```python
from build123d import *

# Parameters (mm, degrees)
BOSS_EXTRUDE1_DEPTH                           = 30
SKETCH2_R                                     = 3.2639
CUT_EXTRUDE1_DEPTH                            = 36
CBORE_FOR_1_4_SOCKET_HEAD_CAP_SCREW1_AT_COUNT = 2
CBORE_FOR_1_4_SOCKET_HEAD_CAP_SCREW1_AT_PITCH = 35
SKETCH7_W                                     = 15
SKETCH7_H                                     = 6.5
BOSS_EXTRUDE2_DEPTH                           = 3
FILLET1_R                                     = 2
CHAMFER1_SIZE                                 = 0.2


with BuildPart() as part:
    # Sketch1 → Boss-Extrude1 (new body)
    with BuildSketch(Plane.XY):
        Polygon((20, 0), (0, 0), (0, 50.45), (-15, 50.45), (-15, 0), (-35, 0), (-35, -20), (20, -20), align=None)
    extrude(amount=BOSS_EXTRUDE1_DEPTH)

    # Sketch2 → Cut-Extrude1 (cut, through all)
    with BuildSketch(Plane(origin=(0, 0, 0), x_dir=(0, 0, -1), z_dir=(1, 0, 0))):
        with Locations((-15, 40.45)):
            Circle(SKETCH2_R)
    extrude(amount=-CUT_EXTRUDE1_DEPTH, mode=Mode.SUBTRACT)

    # Sketch5 → CBORE for 1/4 Socket Head Cap Screw1 (revolve, cut)
    with BuildSketch(Plane(origin=(-25, 0, 15), x_dir=(0, 0, 1), z_dir=(1, 0, 0))):
        Polygon((0, 0), (0, 20), (3.8989, 20), (3.2639, 19.365), (3.2639, 7.984998), (3.8989, 7.349998), (5.55625, 7.349998), (5.55625, 0.635), (6.19125, 0), align=None)
    cbore_for_1_4_socket_head_cap_screw1 = revolve(axis=Axis((-25, 6.35, 15), (0, -1, 0)), mode=Mode.SUBTRACT)

    # CBORE for 1/4 Socket Head Cap Screw1 at: CBORE for 1/4 Socket Head Cap Screw1 ×2
    with Locations(*[(i * CBORE_FOR_1_4_SOCKET_HEAD_CAP_SCREW1_AT_PITCH, 0, 0) for i in range(1, CBORE_FOR_1_4_SOCKET_HEAD_CAP_SCREW1_AT_COUNT)]):
        add(cbore_for_1_4_socket_head_cap_screw1, mode=Mode.SUBTRACT)

    # Sketch7 → Boss-Extrude2 (add)
    with BuildSketch(Plane.XZ.offset(20)):
        with Locations((-7.5, 15)):
            Rectangle(SKETCH7_W, SKETCH7_H)
    extrude(amount=BOSS_EXTRUDE2_DEPTH)

    # Fillet1
    fillet1_edges = [part.edges().sort_by_distance(p)[0] for p in [
        (-35, -10, 30),
        (-15, 25.225, 0),
        (-7.5, 50.45, 0),
        (0, 25.225, 0),
        (10, 0, 0),
        (20, -10, 0),
        (-35, -10, 0),
        (-25, 0, 0),
        (-15, 50.45, 15),
        (0, 50.45, 15),
        (20, 0, 15),
        (-35, 0, 15),
        (20, -10, 30),
        (10, 0, 30),
        (0, 25.225, 30),
        (-7.5, 50.45, 30),
        (-15, 25.225, 30),
        (-25, 0, 30),
        (-15, -21.5, 11.75),
        (0, -21.5, 11.75),
        (0, -21.5, 18.25),
        (-15, -21.5, 18.25),
    ]]
    fillet(fillet1_edges, radius=FILLET1_R)

    # Chamfer1
    chamfer1_edges = [part.edges().sort_by_distance(p)[0] for p in [
        (-35, -20, 15),
        (-34.414213562, -20, 29.414213562),
        (-34.414213562, -20, 0.585786438),
        (19.414213562, -20, 0.585786438),
        (19.414213562, -20, 29.414213562),
        (-15, 40.45, 18.2639),
        (0, 40.45, 18.2639),
        (0, -23, 15),
        (-7.5, -23, 11.75),
        (-7.5, -23, 18.25),
        (-15, -23, 15),
        (-14.414213562, -23, 12.335786438),
        (-14.414213562, -23, 17.664213562),
        (-0.585786438, -23, 17.664213562),
        (-0.585786438, -23, 12.335786438),
        (-7.5, -20, 0),
        (-7.5, -20, 30),
        (20, -20, 15),
    ]]
    chamfer(chamfer1_edges, length=CHAMFER1_SIZE)


solid = part.part
```
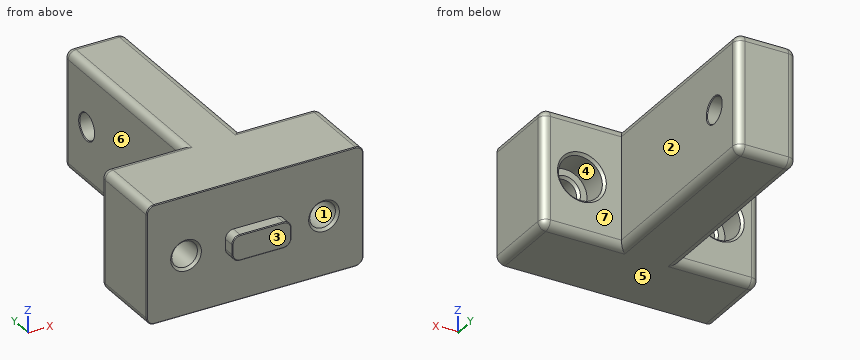
Verification items for the finished model (mm, model axes). Face numbers are marked on the shaded views. A direction names the side the tool comes from. Give positions to 0.01 mm unless a question says otherwise; leave off trailing zeros. Order: outer loops, then holes, each group sorted by start corner. A loop starts at its lowest first (then second) coordinate and runs counter-clockwise, first axis right, second up. Notation, with made-up numbers: (54.25, 74.25) -> (90.25, 74.25) arc R10 cw to (90.25, 90.25) -> close; hole circle Ø5 at (64, 25). An arc over 180 degrees is marked (long way). Use a Markdown table: item, result.
1) Section check C-C, the plane x = -17.5. Record the boundary of the cut face in (y, z), then the cut area to 3 significant figures.
Results:
| item | result |
|---|---|
| outline | (-20, 0.2) -> (-19.8, 0) -> (-2, 0) arc R2 ccw to (0, 2) -> (0, 28) arc R2 ccw to (-2, 30) -> (-19.8, 30) -> (-20, 29.8) -> close |
| area | 598 mm² |
2) Material ranges on probe 1 along X at (y, z) = (-3.5, 15); probe 2 along X at (y, z) = (-11, 14.75); probe 3 along Z at (x, y) = (10, -3), recorded low to high.
Results:
| item | result |
|---|---|
| probe 1 | -35 to -30.56, -19.44 to 4.44, 15.56 to 20 |
| probe 2 | -35 to -28.25, -21.75 to 6.75, 13.25 to 20 |
| probe 3 | 0 to 9.44, 20.56 to 30 |
3) Mould release check, pull along X, two halves, no side actions. Record for the marked faces 1, 2 and 3: pulls with the +X half, pulls with the -X half, needs draft (parallel to the pull), parting line crosses it, or undercut.
Results:
| item | result |
|---|---|
| face 1 | undercut |
| face 2 | pulls with the +X half |
| face 3 | needs draft |
4) Section check A-A, the plane x = -25. Record the boundary of the cut face in (y, z) (3 decimals).
Results:
| item | result |
|---|---|
| outline | (-20, 0.2) -> (-19.8, 0) -> (-2, 0) arc R2 ccw to (0, 2) -> (0, 8.809) -> (-0.635, 9.444) -> (-7.35, 9.444) -> (-7.35, 11.101) -> (-7.985, 11.736) -> (-19.365, 11.736) -> (-20, 11.101) -> close; (-20, 18.899) -> (-19.365, 18.264) -> (-7.985, 18.264) -> (-7.35, 18.899) -> (-7.35, 20.556) -> (-0.635, 20.556) -> (0, 21.191) -> (0, 28) arc R2 ccw to (-2, 30) -> (-19.8, 30) -> (-20, 29.8) -> close |
5) Section check B-B, the plane y = 40.45. Record the boundary of the cut face in (x, z).
Results:
| item | result |
|---|---|
| outline | (-15, 2) arc R2 ccw to (-13, 0) -> (-2, 0) arc R2 ccw to (0, 2) -> (0, 11.54) -> (-0.2, 11.74) -> (-14.8, 11.74) -> (-15, 11.54) -> close; (-15, 18.46) -> (-14.8, 18.26) -> (-0.2, 18.26) -> (0, 18.46) -> (0, 28) arc R2 ccw to (-2, 30) -> (-13, 30) arc R2 ccw to (-15, 28) -> close |
6) Depth check by flat-ended pin: pin 1 Ø3 at (x, z) = (-27, 24.5) entering from -Y; pin 2 Ø3 at (y, z) = (32, 21) entering from +X; pin 3 Ø12 at (x, z) = (-27.5, 15) entering from +Y. Enter the tip coordinate at first touch or a pass-through.
Results:
| item | result |
|---|---|
| pin 1 | y = -20 |
| pin 2 | x = 0 |
| pin 3 | y = 0 |
7) Tool access check on the marked faces 4, 5, 6 and 7. Record the directions out of +Z, -Z, +X, -X, +Y, -Y that give a thin tool (end or side, any length) a straight path to the whole face; none if there is none.
Results:
| item | result |
|---|---|
| face 4 | +Y |
| face 5 | -Z, +X, -X, +Y, -Y |
| face 6 | +Z, -Z, -X, +Y |
| face 7 | +Z, -Z, +X, +Y |
8) Section check D-D, the plane y = -11.5. Record the boundary of the cut face in (x, z).
Results:
| item | result |
|---|---|
| outline | (-35, 2) arc R2 ccw to (-33, 0) -> (18, 0) arc R2 ccw to (20, 2) -> (20, 28) arc R2 ccw to (18, 30) -> (-33, 30) arc R2 ccw to (-35, 28) -> close; hole circle Ø6.53 at (-25, 15); hole circle Ø6.53 at (10, 15) |
